Work out the finished part from the listing and answer in its coordinate system (mm). A direction names the side the tool comes from. Coordinates: 2 decimals unless noted, no trailing zeros. Answer as CSV lines item,"result". Start each with the question number.
(1) For faces 1 (the flat face through (-85, 92, 20)), 2 (the flat face through (-42.447, 92, 31)), 3 (the flat face through (-68.447, 93, 45)), 4 (the cylindrical face through (-55.8, 104.5, 45.5)), 5 (the cylindrical face through (0.66, 9.86, 14.985)), determine the directions among +Z, -Z, +X, -X, +Y, -Y from which every point of the face is accessible in a straight line to the end or side of a thin tool.
(2) A cutting plane is placed at A-A on z = 38.5. Count the separate pieces of the cut face and the enclosed holes in it, then the cut area to 3 significant figures.
(3) The mould has two halves that part along Y. Classify faces 6 (the cylindrical face through (-208.357, 195.871, 0.28)), 7 (the cylindrical face through (-112.919, 77.275, 0.28)), 8 (the flat face through (-150, 160, 47)): released by +Y, released by -Y, zero draft, split by the parting line, or undercut.
(4) Find the intervals of material crossed by L1, parallel to Y at x = 9.5, z = 23.5; L2, parallel to Y at x = 69.5, z = 18; L3, parallel to Y at x = -150, z = -4.75, in increasing order. Write a range as [from, to].
(5) Flat-ended cylindrical pins translate along their axes: P1, Ø24, axis at x = -144.5, y = 157, coming from the -Z side; P2, Ø9.5, axis at y = 91.5, z = 35.5, coming from the +X side; P3, Ø6.5, axis at x = -84, y = 91.5, coming from the +Z side; P4, Ø8, axis at y = 85, z = -26, coming from the +X side. Find the tip coordinate at first contact, or state that the pin passes through.
from build123d import *

# Parameters (mm, degrees)
SKETCH1_R            = 90
BOSS_EXTRUDE1_DEPTH  = 37
CHAMFER1_SIZE        = 6
SKETCH2_W            = 155
SKETCH2_H            = 40
BOSS_EXTRUDE2_DEPTH  = 50
CUT_EXTRUDE1_DEPTH   = 40
BOSS_EXTRUDE3_DEPTH  = 20
SKETCH8_R            = 50
BOSS_EXTRUDE4_DEPTH  = 3
SKETCH12_R           = 20
BOSS_EXTRUDE5_DEPTH  = 2
BOSS_EXTRUDE6_DEPTH  = 1
SKETCH14_R           = 9.5
BOSS_EXTRUDE7_DEPTH  = 2
BOSS_EXTRUDE9_DEPTH  = 22
BOSS_EXTRUDE10_DEPTH = 7
SKETCH18_R           = 6.5
BOSS_EXTRUDE11_DEPTH = 1
SKETCH19_R           = 21
SKETCH19_R_2         = 20
CUT_EXTRUDE12_DEPTH  = 0.1
FILLET1_R            = 2
SKETCH20_R           = 15
CUT_EXTRUDE13_DEPTH  = 20
SKETCH21_R           = 15
CUT_EXTRUDE14_DEPTH  = 20


with BuildPart() as part:
    # Sketch1 → Boss-Extrude1 (new body)
    with BuildSketch(Plane(origin=(0, 0, 0), x_dir=(1, 0, 0), z_dir=(0, 1, 0))):
        with Locations(Location((0, 0, 0), (0, 0, 270))):
            Circle(SKETCH1_R)
    extrude(amount=BOSS_EXTRUDE1_DEPTH)

    # Chamfer1
    chamfer1_edges = [part.edges().sort_by_distance(p)[0] for p in [
        (0, 37, -90),
    ]]
    chamfer(chamfer1_edges, length=CHAMFER1_SIZE)

    # Sketch2 → Boss-Extrude2 (add)
    with BuildSketch(Plane(origin=(0, 37, 0), x_dir=(1, 0, 0), z_dir=(0, 1, 0))):
        Rectangle(SKETCH2_W, SKETCH2_H)
    extrude(amount=BOSS_EXTRUDE2_DEPTH)

    # Sketch3 → Cut-Extrude1 (cut)
    with BuildSketch(Plane.XY.offset(20)):
        with BuildLine():
            Line((-77.5, 48), (-77.5, 87))
            Line((-77.5, 87), (32.5, 87))
            ThreePointArc((32.5, 87), (-18.551432041, 56.363013449), (-77.5, 48))
        make_face()
    extrude(amount=-CUT_EXTRUDE1_DEPTH, mode=Mode.SUBTRACT)

    # Sketch4 → Boss-Extrude3 (add, symmetric)
    with BuildSketch(Plane.XY):
        with BuildLine():
            ThreePointArc((-95.279461367, 201.205735666), (-209.325156185, 194.245814981), (-158.315351417, 92.00658171))
            ThreePointArc((-158.315351417, 92.00658171), (-113.710864551, 77.710473629), (-77.5, 48))
            ThreePointArc((-77.5, 48), (-18.551432041, 56.363013449), (32.5, 87))
            ThreePointArc((32.5, 87), (-37.003814726, 137.821531516), (-95.279461367, 201.205735666))
        make_face()
    extrude(amount=BOSS_EXTRUDE3_DEPTH, both=True)

    # Sketch8 → Boss-Extrude4 (add)
    with BuildSketch(Plane.XY.offset(20)):
        with Locations(Location((-150, 160, 0), (0, 0, 180))):
            Circle(SKETCH8_R)
    extrude(amount=BOSS_EXTRUDE4_DEPTH)

    # Loft2: read off the stored shape, not the designer's step
    # Loft2: loft between two sections, ruled curve by curve
    loft2_from = [
        Edge.make_bspline([(-197.405095184, 175.898331692, 23), (-229.201758567, 81.088141323, 23), (-134.391568199, 49.29147794, 23), (-102.594904816, 144.101668308, 23), (-70.798241433, 238.911858677, 23), (-165.608431801, 270.70852206, 23), (-197.405095184, 175.898331692, 23)], [0, 0, 0, 0, 0.5, 0.5, 0.5, 1, 1, 1, 1], 3, [1, 0.333333333, 0.333333333, 1, 0.333333333, 0.333333333, 1]),
    ]
    loft2_to = [
        Edge.make_bspline([(-179.935973003, 158.041041, 42), (-176.018055003, 98.169094994, 42), (-116.146108997, 102.087012994, 42), (-120.064026997, 161.958959, 42), (-123.981944997, 221.830905006, 42), (-183.853891003, 217.912987006, 42), (-179.935973003, 158.041041, 42)], [0, 0, 0, 0, 0.5, 0.5, 0.5, 1, 1, 1, 1], 3, [1, 0.333333333, 0.333333333, 1, 0.333333333, 0.333333333, 1]),
    ]
    loft2 = Solid(Shell([*[Face.make_surface_from_curves(loft2_from[k], loft2_to[k]) for k in range(1)], Face(Wire(loft2_from)), Face(Wire(loft2_to))]))
    add(loft2)

    # Sketch12 → Boss-Extrude5 (add)
    with BuildSketch(Plane.XY.offset(42)):
        with Locations((-150, 160)):
            Circle(SKETCH12_R)
    extrude(amount=BOSS_EXTRUDE5_DEPTH)

    # Sketch13 → Boss-Extrude6 (add)
    with BuildSketch(Plane.XY.offset(44)):
        with BuildLine():
            Line((-154.973420243, 179.371760144), (-152.561527516, 172.74513934))
            ThreePointArc((-152.561527516, 172.74513934), (-159.168635276, 169.216079816), (-162.73174885, 162.627274483))
            Line((-162.73174885, 162.627274483), (-169.355073812, 165.037967621))
            ThreePointArc((-169.355073812, 165.037967621), (-170, 160), (-169.355073812, 154.962032379))
            Line((-169.355073812, 154.962032379), (-162.73174885, 157.372725517))
            ThreePointArc((-162.73174885, 157.372725517), (-158.958779481, 150.579794577), (-151.985076295, 147.152452681))
            Line((-151.985076295, 147.152452681), (-154.409249727, 140.492090916))
            ThreePointArc((-154.409249727, 140.492090916), (-150, 140), (-145.590750273, 140.492090916))
            Line((-145.590750273, 140.492090916), (-148.014923705, 147.152452681))
            ThreePointArc((-148.014923705, 147.152452681), (-141.101752828, 150.522595436), (-137.302957602, 157.209818223))
            Line((-137.302957602, 157.209818223), (-130.687310868, 154.801919732))
            ThreePointArc((-130.687310868, 154.801919732), (-130.172572246, 157.378338566), (-130, 160))
            ThreePointArc((-130, 160), (-130.172572246, 162.621661434), (-130.687310868, 165.198080268))
            Line((-130.687310868, 165.198080268), (-137.302957602, 162.790181777))
            ThreePointArc((-137.302957602, 162.790181777), (-140.890593654, 169.274627541), (-147.438472484, 172.74513934))
            Line((-147.438472484, 172.74513934), (-145.026579757, 179.371760144))
            ThreePointArc((-145.026579757, 179.371760144), (-150, 180), (-154.973420243, 179.371760144))
        make_face()
    extrude(amount=BOSS_EXTRUDE6_DEPTH)

    # Sketch14 → Boss-Extrude7 (add)
    with BuildSketch(Plane.XY.offset(45)):
        with Locations((-150, 160)):
            Circle(SKETCH14_R)
    extrude(amount=BOSS_EXTRUDE7_DEPTH)

    # Sketch16 → Boss-Extrude9 (add)
    with BuildSketch(Plane.XY.offset(20)):
        with BuildLine():
            Line((-69.446792895, 101.883912358), (-69.446792895, 82.883912358))
            ThreePointArc((-69.446792895, 82.883912358), (-55.946792895, 79.266598261), (-42.446792895, 82.883912358))
            Line((-42.446792895, 82.883912358), (-42.446792895, 101.883912358))
            ThreePointArc((-42.446792895, 101.883912358), (-55.946792895, 105.501226456), (-69.446792895, 101.883912358))
        make_face()
    extrude(amount=BOSS_EXTRUDE9_DEPTH)

    # Sketch17 → Boss-Extrude10 (add)
    with BuildSketch(Plane.XY.offset(42)):
        with BuildLine():
            Line((-43.446792895, 83.46857203), (-43.446792895, 101.299252687))
            ThreePointArc((-43.446792895, 101.299252687), (-55.946792895, 104.501226456), (-68.446792895, 101.299252687))
            Line((-68.446792895, 101.299252687), (-68.446792895, 83.46857203))
            ThreePointArc((-68.446792895, 83.46857203), (-55.946792895, 80.266598261), (-43.446792895, 83.46857203))
        make_face()
    extrude(amount=BOSS_EXTRUDE10_DEPTH)

    # Sketch18 → Boss-Extrude11 (add)
    with BuildSketch(Plane.XY.offset(20)):
        Polygon((-84.446792895, 83.146308051), (-76.446792895, 87.765110205), (-76.446792895, 97.002714512), (-84.446792895, 101.621516665), (-92.446792895, 97.002714512), (-92.446792895, 87.765110205), align=None)
        with Locations((-84.446792895, 92.383912358)):
            Circle(SKETCH18_R, mode=Mode.SUBTRACT)
    extrude(amount=BOSS_EXTRUDE11_DEPTH)

    # Sketch19 → Cut-Extrude12 (cut)
    with BuildSketch(Plane.XY.offset(20)):
        with Locations((-55.946792895, 92.383912358)):
            Circle(SKETCH19_R)
        with Locations((-55.946792895, 92.383912358)):
            Circle(SKETCH19_R_2, mode=Mode.SUBTRACT)
    extrude(amount=-CUT_EXTRUDE12_DEPTH, mode=Mode.SUBTRACT)

    # Fillet1
    fillet1_edges = [part.edges().sort_by_distance(p)[0] for p in [
        (77.5, 62, 20),
        (77.5, 62, -20),
        (77.5, 87, 0),
        (55, 87, -20),
        (55, 87, 20),
        (-77.5, 42.5, 20),
        (-77.5, 42.5, -20),
        (0, 37, -84),
    ]]
    fillet(fillet1_edges, radius=FILLET1_R)

    # Sketch20 → Cut-Extrude13 (cut)
    with BuildSketch(Plane.XZ):
        with Locations(Location((0, 0, 0), (0, 0, 270))):
            Circle(SKETCH20_R)
    extrude(amount=-CUT_EXTRUDE13_DEPTH, mode=Mode.SUBTRACT)

    # Sketch21 → Cut-Extrude14 (cut)
    with BuildSketch(Plane(origin=(0, 0, -20), x_dir=(-1, 0, 0), z_dir=(0, 0, -1))):
        with Locations((150, 160)):
            Circle(SKETCH21_R)
    extrude(amount=-CUT_EXTRUDE14_DEPTH, mode=Mode.SUBTRACT)


solid = part.part
Here are the results:
1,face 1,"+Z"
1,face 2,"+Z, +X, +Y"
1,face 3,"+Z, -X, +Y"
1,face 4,"+Z, +Y"
1,face 5,"-Y"
2,separate pieces,"3"
2,enclosed holes,"0"
2,area,"10,100 mm^2"
3,face 6,"split by the parting line"
3,face 7,"undercut"
3,face 8,"zero draft"
4,L1,"y = [0, 37]"
4,L2,"y = [0, 87]"
4,L3,"y = [90.7, 145], [175, 228.5]"
5,P1,"stops at z = -20"
5,P2,"stops at x = -42.45"
5,P3,"stops at z = 20"
5,P4,"passes through"
